Can you work these out from the model? Positions are in its coordinate system, mm. Give positions to 0.01 mm unless a question says otherwise; leave off trailing zeros. Order: outer loops, then holes, each group sorted by start corner. A loop starts at its lowest first (then second) coordinate and runs counter-clockwise, first axis right, second up. Notation, with made-up numbers: M -2,-28 L 11,-28 A33 cw 11,6 Z; hole C 80.25,30.5 d11. An arc over 180 degrees is marked long. Use one line per item in the form item = value. Start each with the question number.
1. Will this pin go through, and if not, where does the flat tip stop? P1, Ø8, axis at x = 33, y = -5.5, coming from the +Z side.
2. I want a section at B-B, the plane x = -27. List the corners of the cut face in (y, z) for me.
3. I need wall thicknesses on L1, parallel to X at y = 6.5, z = 1.35; L2, parallel to X at y = 0, z = 1.4; L3, parallel to Y at x = 38.5, z = 0.7. Which ranges of each line are inside material? Lowest first, please.
4. I want a section at A-A, the plane y = -19. List the corners of the cut face in (x, z) for me, and give its area (3 significant figures).
5. I want a section at D-D, the plane y = 17. List the corners of the cut face in (x, z) for me, and give its area (3 significant figures).
6. I want a section at C-C, the plane z = 2.1. Count the separate pieces of the cut face and the enclosed holes in it, and give its area (3 significant figures).
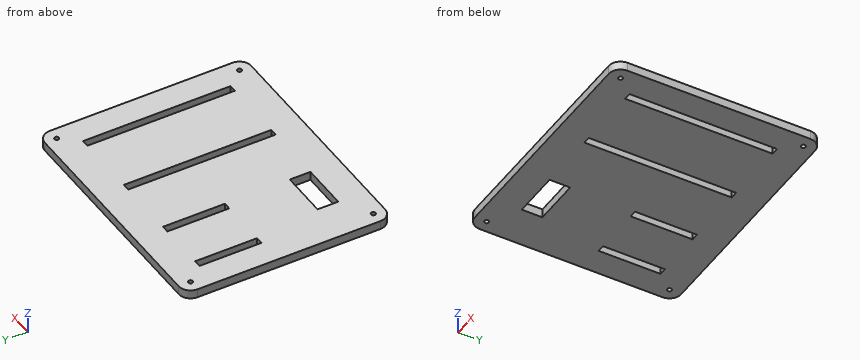
```python
from build123d import *

# Parameters (mm, degrees)
SKETCH1_W           = 85
SKETCH1_H           = 70
BOSS_EXTRUDE1_DEPTH = 3
SKETCH2_W           = 2.5
SKETCH2_H           = 50
SKETCH2_H_2         = 21
SKETCH2_W_2         = 16
SKETCH2_H_3         = 7
CUT_EXTRUDE1_DEPTH  = 56.138462075
FILLET1_R           = 4
SKETCH4_R           = 0.75
CUT_EXTRUDE3_DEPTH  = 10


with BuildPart() as part:
    # Sketch1 → Boss-Extrude1 (new body)
    with BuildSketch(Plane.XY):
        Rectangle(SKETCH1_W, SKETCH1_H)
    extrude(amount=BOSS_EXTRUDE1_DEPTH)

    # Sketch2 → Cut-Extrude1 (cut, through all)
    with BuildSketch(Plane(origin=(0, 0, 0), x_dir=(-1, 0, 0), z_dir=(0, 0, -1))):
        with Locations((-32.25, 0)):
            Rectangle(SKETCH2_W, SKETCH2_H)
        with Locations((-8.75, 0)):
            Rectangle(SKETCH2_W, SKETCH2_H)
        with Locations((13.75, 14.5)):
            Rectangle(SKETCH2_W, SKETCH2_H_2)
        with Locations((32.25, 14.5)):
            Rectangle(SKETCH2_W, SKETCH2_H_2)
        with Locations((20.5, -21.5)):
            Rectangle(SKETCH2_W_2, SKETCH2_H_3)
    extrude(amount=-CUT_EXTRUDE1_DEPTH, mode=Mode.SUBTRACT)

    # Fillet1
    fillet1_edges = [part.edges().sort_by_distance(p)[0] for p in [
        (42.5, -35, 1.5),
        (-42.5, -35, 1.5),
        (-42.5, 35, 1.5),
        (42.5, 35, 1.5),
    ]]
    fillet(fillet1_edges, radius=FILLET1_R)

    # Sketch4 → Cut-Extrude3 (cut)
    with BuildSketch(Plane(origin=(0, 0, 0), x_dir=(-1, 0, 0), z_dir=(0, 0, -1))):
        with Locations((-38.5, 31)):
            Circle(SKETCH4_R)
        with Locations(Location((38.5, 31, 0), (0, 0, 180))):
            Circle(SKETCH4_R)
        with Locations((38.5, -31)):
            Circle(SKETCH4_R)
        with Locations(Location((-38.5, -31, 0), (0, 0, 180))):
            Circle(SKETCH4_R)
    extrude(amount=-CUT_EXTRUDE3_DEPTH, mode=Mode.SUBTRACT)


solid = part.part
```
Check result:
q1.P1 = 3
q2.outline = M -35,0 L -25,0 L -25,3 L -35,3 Z; M -18,0 L 35,0 L 35,3 L -18,3 Z
q3.L1 = -42.5 to -33.5, -31 to -15, -12.5 to 7.5, 10 to 31, 33.5 to 42.5
q3.L2 = -42.5 to 7.5, 10 to 31, 33.5 to 42.5
q3.L3 = -35 to -31.75, -30.25 to 30.25, 31.75 to 35
q4.outline = M -42.5,0 L -28.5,0 L -28.5,3 L -42.5,3 Z; M -12.5,0 L 7.5,0 L 7.5,3 L -12.5,3 Z; M 10,0 L 31,0 L 31,3 L 10,3 Z; M 33.5,0 L 42.5,0 L 42.5,3 L 33.5,3 Z
q4.area = 192 mm2
q5.outline = M -42.5,0 L -33.5,0 L -33.5,3 L -42.5,3 Z; M -31,0 L -15,0 L -15,3 L -31,3 Z; M -12.5,0 L 7.5,0 L 7.5,3 L -12.5,3 Z; M 10,0 L 31,0 L 31,3 L 10,3 Z; M 33.5,0 L 42.5,0 L 42.5,3 L 33.5,3 Z
q5.area = 225 mm2
q6.separate_pieces = 1
q6.enclosed_holes = 9
q6.area = 5,460 mm2
